Build history of the part. All positions in model axes, mm. A direction names the side the tool comes from. Give positions to 0.01 mm unless a question says otherwise; leave off trailing zeros. Loops run counter-clockwise (first coordinate to the right, second up) from the corner with the lowest first, then second, coordinate; pieces in that order, holes last. Notation, with made-up numbers: M 34.5,-23 L 57.5,-23 A21 cw 57.5,9 Z; hole C -9.5,-9 d2. An arc over 180 degrees is marked long. Put each result on its own line as item: value.
```python
from build123d import *

# Parameters (mm, degrees)
F1_DEPTH = 10


with BuildPart() as f1:
    # F0 (on Top) → F1 (new body)
    with BuildSketch(Plane.XY):
        with BuildLine():
            ThreePointArc((-24.958041373, 39.2821468413), (-25.4915434809, 41.3805095925), (-25.8489488203, 43.5159280896))
            Line((-25.8489488203, 43.5159280896), (-31.9847488633, 43.5159280896))
            ThreePointArc((-31.9847488633, 43.5159280896), (-31.6977160516, 41.3870765544), (-31.2691514741, 39.2821468413))
            Line((-31.2691514741, 39.2821468413), (-24.958041373, 39.2821468413))
        make_face()
        with BuildLine():
            Line((35.0935831666, 39.2821468413), (31.2691514741, 39.2821468413))
            ThreePointArc((31.2691514741, 39.2821468413), (0, 14.5973533174), (-31.2691514741, 39.2821468413))
            Line((-31.2691514741, 39.2821468413), (-35.0935831666, 39.2821468413))
            Line((-35.0935831666, 39.2821468413), (-35.0935831666, -46.7446520925))
            Line((-35.0935831666, -46.7446520925), (35.0935831666, -46.7446520925))
            Line((35.0935831666, -46.7446520925), (35.0935831666, 39.2821468413))
        make_face()
        with BuildLine():
            ThreePointArc((-31.2691514741, 39.2821468413), (-31.6977160516, 41.3870765544), (-31.9847488633, 43.5159280896))
            Line((-31.9847488633, 43.5159280896), (-35.0935831666, 43.5159280896))
            Line((-35.0935831666, 43.5159280896), (-35.0935831666, 39.2821468413))
            Line((-35.0935831666, 39.2821468413), (-31.2691514741, 39.2821468413))
        make_face()
        with BuildLine():
            ThreePointArc((24.958041373, 39.2821468413), (25.4915434809, 41.3805095925), (25.8489488203, 43.5159280896))
            Line((25.8489488203, 43.5159280896), (-25.8489488203, 43.5159280896))
            ThreePointArc((-25.8489488203, 43.5159280896), (-25.4915434809, 41.3805095925), (-24.958041373, 39.2821468413))
            Line((-24.958041373, 39.2821468413), (24.958041373, 39.2821468413))
        make_face()
        with BuildLine():
            Line((31.9847488633, 43.5159280896), (25.8489488203, 43.5159280896))
            ThreePointArc((25.8489488203, 43.5159280896), (25.4915434809, 41.3805095925), (24.958041373, 39.2821468413))
            Line((24.958041373, 39.2821468413), (31.2691514741, 39.2821468413))
            ThreePointArc((31.2691514741, 39.2821468413), (31.6977160516, 41.3870765544), (31.9847488633, 43.5159280896))
        make_face()
        with BuildLine():
            Line((35.0935831666, 43.5159280896), (31.9847488633, 43.5159280896))
            ThreePointArc((31.9847488633, 43.5159280896), (31.6977160516, 41.3870765544), (31.2691514741, 39.2821468413))
            Line((31.2691514741, 39.2821468413), (35.0935831666, 39.2821468413))
            Line((35.0935831666, 39.2821468413), (35.0935831666, 43.5159280896))
        make_face()
        with BuildLine():
            ThreePointArc((-24.958041373, 39.2821468413), (0, 20.6948380086), (24.958041373, 39.2821468413))
            Line((24.958041373, 39.2821468413), (-24.958041373, 39.2821468413))
        make_face()
    extrude(amount=F1_DEPTH)


solid = f1.part
```
Q1. Slice it at B-B (x = 0). List the corners of the cut face in (y, z).
Here are the results:
outline: M -46.74,0 L 14.6,0 L 14.6,10 L -46.74,10 Z; M 20.69,0 L 43.52,0 L 43.52,10 L 20.69,10 Z
Q2. Probe line 1 (X direction, y = 19, z = 5.5); line 2 (Y direction, x = 10, z = 5.75); line 3 (Y direction, x = -7.5, z = 4). List the from-to ranges inside material, lowest first. Write a range as from..to.
Here are the results:
line 1: -35.09..-16.24, 16.24..35.09
line 2: -46.74..16.19, 22.69..43.52
line 3: -46.74..15.48, 21.8..43.52
Q3. Slice it at A-A (z = 2.5). List the corners of the cut face in (x, y), and give its area (3 significant figures).
Here are the results:
outline: M -35.09,-46.74 L 35.09,-46.74 L 35.09,43.52 L -35.09,43.52 Z; hole M -31.27,39.28 A32.15 ccw 31.27,39.28 L 24.96,39.28 A26.05 cw -24.96,39.28 Z
area: 5,870 mm²
Q4. Mould opens along Y. For faces 1 (the flat face through (0, 43.516, 5)), 2 (the flat face through (35.094, -2, 5)), 3 (the flat face through (28, 39.282, 5)) say: pulls with the +Y half, pulls with the -Y half, needs draft (parallel to the pull), parting line crosses it, or undercut.
Here are the results:
face 1: pulls with the +Y half
face 2: needs draft
face 3: undercut
Q5. Tool access for faces 4 (the flat face through (0, -1, 0)), 5 (the cylindrical face through (-0.5, 20.7, 4.9)): list every direction of +Z, -Z, +X, -X, +Y, -Y with a clear straight run to the whole face (end or side of a thin tool).
Here are the results:
face 4: -Z, +X, -X, +Y, -Y
face 5: +Z, -Z
Q6. Slice it at C-C (y = 24). List the corners of the cut face in (x, z).
Here are the results:
outline: M -35.09,0 L -22.72,0 L -22.72,10 L -35.09,10 Z; M -12.7,0 L 12.7,0 L 12.7,10 L -12.7,10 Z; M 22.72,0 L 35.09,0 L 35.09,10 L 22.72,10 Z
Q7. Slice it at D-D (x = 14). List the corners of the cut face in (y, z), and give its area (3 significant figures).
Here are the results:
outline: M -46.74,0 L 17.81,0 L 17.81,10 L -46.74,10 Z; M 24.78,0 L 43.52,0 L 43.52,10 L 24.78,10 Z
area: 833 mm²
